Geometry: see drawing. Coordinates: mm, zero at the bounding-box minimum. A direction names the side the tool comes from. Round coordinates to 2 decimals unless told otherwise and drop trailing zeros. Loops run counter-clockwise (first coordinate to the right, second up) from the corner with the lowest first, then second, coordinate; pieces in that order, holes last. Notation, with made-up numbers: (47.5, 59) - (99.5, 59) arc R23 ccw to (99.5, 96) - close; hole circle Ø5 at (-32.5, 47). An arc over 180 degrees is marked (long way). Return JSON: item names as keys, results as strings. Group by question number.
1. Section A-A on y = 1.1. Return loops of the section in (x, z), and give its area (3 significant figures).
2. Set-up query: the marked faces 1 and 2. Return all of +Z, -Z, +X, -X, +Y, -Y with unobstructed straight access to the full face (end or side cutting, diameter ignored); none if empty.
3. Section B-B on y = 1.7. Return loops of the section in (x, z), and give its area (3 significant figures).
4. Section C-C on x = 7.25. Return loops of the section in (y, z), and give its area (3 significant figures).
5. Section D-D on y = 2.7. Return loops of the section in (x, z).
6. First-contact query: pin 1 Ø0.7 at (x, z) = (10.5, 6.5) entering from +Y; pin 2 Ø1.1 at (y, z) = (1.5, 4) entering from -X. Flat tips, straight axial feed; report the tip coordinate or a pass-through.
7. Material intervals for probe 1 along X at (y, z) = (0.35, 7.75); probe 2 along Z at (x, y) = (10.35, 1.1); probe 3 along Z at (x, y) = (3, 1.8), sorted ascending.
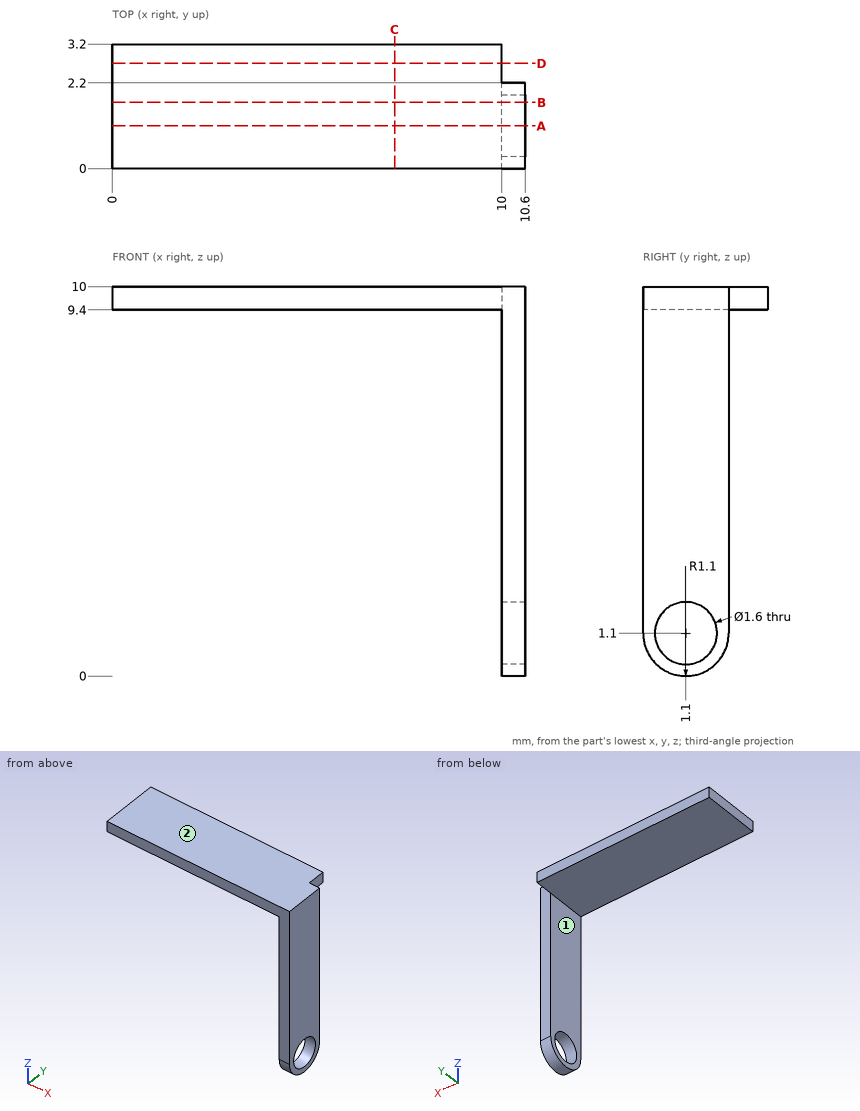
Taken from the geometry:
{
 "1": {"outline": "(0, 9.4) - (10, 9.4) - (10, 1.9) - (10.6, 1.9) - (10.6, 10) - (0, 10) - close; (10, 0) - (10.6, 0) - (10.6, 0.3) - (10, 0.3) - close", "area": "11.0 mm2"},
 "2": {"face 1": "-Z, -X, +Y, -Y", "face 2": "+Z, +X, -X, +Y, -Y"},
 "3": {"outline": "(0, 9.4) - (10, 9.4) - (10, 1.63) - (10.6, 1.63) - (10.6, 10) - (0, 10) - close; (10, 0.18) - (10.6, 0.18) - (10.6, 0.57) - (10, 0.57) - close", "area": "11.3 mm2"},
 "4": {"outline": "(0, 9.4) - (3.2, 9.4) - (3.2, 10) - (0, 10) - close", "area": "1.92 mm2"},
 "5": {"outline": "(0, 9.4) - (10, 9.4) - (10, 10) - (0, 10) - close"},
 "6": {"pin 1": "y = 2.2", "pin 2": "x = 10"},
 "7": {"probe 1": "10 to 10.6", "probe 2": "0 to 0.3, 1.9 to 10", "probe 3": "9.4 to 10"}
}
